Can you work these out from the model? Positions are in its coordinate system, mm. A direction names the side the tool comes from. Coordinates: 2 decimals unless noted, no trailing zeros. Order: outer loops, then holes, each group sorted by start corner. A loop starts at its lowest first (then second) coordinate and runs counter-clockwise, first axis right, second up. Notation, with made-up numbers: (-11.5, 48.5) -> (-6.5, 48.5) arc R13 cw to (-6.5, 58.5) -> close; hole circle Ø3 at (13, 6). An arc over 180 degrees is marked (long way). Answer as CSV lines item,"result".
Autodesk Inventor part; units mm, degrees
ref_plane "YZ Plane" through (0, 0, 0) normal (1, 0, 0) x (0, 1, 0)
ref_plane "XZ Plane" through (0, 0, 0) normal (0, 1, 0) x (-1, 0, 0)
ref_plane "XY Plane" through (0, 0, 0) normal (0, 0, 1) x (1, 0, 0)
sketch "Sketch1" plane through (0, 0, 0) normal (0, 1, 0) x (-1, 0, 0)
  line L0 (0, 0) -> (28, 0)
  line L1 (28, 0) -> (28, -6)
  line L2 (28, -6) -> (0, -6)
  line L3 (0, -6) -> (0, 0)
  dimension "d0" = 28
  dimension "d1" = 6
extrude "Extrusion1" add sketch "Sketch1" along normal blind 2.54
hole "Hole1" at (-25.5, 2.54, -2.952) direction (0, -1, 0) diameter 4 end through all
hole "Hole2" at (-2.5, 2.54, -2.952) direction (0, -1, 0) diameter 4 end through all
sketch "Sketch2" plane through (0, 0, 0) normal (1, 0, 0) x (0, 0, -1)
  circle A0 centre (-3.7852, -0.96) radius 3.5
  line L0 (-3.7852, 2.54) -> (0.6598, 2.54)
  line L1 (0, 2.54) -> (6, 2.54)
  line L2 (6, 0) -> (0, 0)
  line L3 (-0.4194, 0) -> (0, 0)
  line L4 (0, 0) -> (-0.4194, 0)
  line L5 (0.2994, 0) -> (-3.7852, 0)
  line L6 (-3.7852, 0) -> (-3.7852, 2.54)
  line L7 (-3.7852, 2.54) -> (0.2994, 2.54)
  line L8 (0.2994, 2.54) -> (0.2994, 0)
  line L9 (0.2994, 2.54) -> (-3.6886, 2.54)
  line L10 (-3.6886, 2.54) -> (-3.6886, 0)
  line L11 (-3.6886, 0) -> (0.2994, 0)
  line L12 (0.2994, 0) -> (0.2994, 2.54)
  dimension "d22" = 7
  dimension "d41" = 4.445
extrude "Extrusion2" add sketch "Sketch2" against normal blind 28
sketch "Sketch3" plane through (0, 2.54, 0) normal (0, 1, 0) x (1, 0, 0)
  line L0 (-28, 0) -> (-17.5, 0)
  line L1 (-17.5, 0) -> (-17.5, -12.7)
  line L2 (-17.5, -12.7) -> (-28, -12.7)
  line L3 (-28, -12.7) -> (-28, 0)
  line L4 (0, 0) -> (0, 6)
  line L5 (0, 0) -> (-10.5, 0)
  line L6 (-10.5, 0) -> (-10.5, -9.3969)
  line L7 (-10.5, -9.3969) -> (0, -9.3969)
  line L8 (0, -9.3969) -> (0, 0)
  dimension "d28" = 7
  dimension "d29" = 10.5
  dimension "d42" = 12.7
extrude "Extrusion3" cut sketch "Sketch3" against normal blind 28
hole "Hole3" at (-10.5, -0.96, 3.7852) direction (-1, 0, 0) diameter 3 end through all
properties part number "camera holderpt2"
Q1. Imagine slicing it at A-A (y = -0.96). List the corners of the cut face in (x, z) for me.
Solution:
outline,"(-17.5, 0.29) -> (-10.5, 0.29) -> (-10.5, 2.29) -> (-17.5, 2.29) -> close; (-17.5, 5.29) -> (-10.5, 5.29) -> (-10.5, 7.29) -> (-17.5, 7.29) -> close"
Q2. Imagine slicing it at C-C (y = 2.25). List the corners of the cut face in (x, z) for me, and give its area (3 significant figures).
Solution:
outline,"(-28, -6) -> (0, -6) -> (0, 0) -> (-10.5, 0) -> (-10.5, 5.18) -> (-17.5, 5.18) -> (-17.5, 0) -> (-28, 0) -> close; hole circle Ø4 at (-25.5, -2.95); hole circle Ø4 at (-2.5, -2.95)"
area,"179 mm2"
Q3. Imagine slicing it at D-D (x = -16). List the corners of the cut face in (y, z) for me, and give its area (3 significant figures).
Solution:
outline,"(0, -6) -> (2.54, -6) -> (2.54, 3.69) arc R3.5 ccw (long way) to (0, 0.42) -> close; hole circle Ø3 at (-0.96, 3.79)"
area,"50.0 mm2"
Q4. If I drill on line 1 (X direction, y = 1.75, z = -3); line 2 (Z direction, x = -2.5, y = 1.8); line 3 (Z direction, x = -21.5, y = 0.75), over which ranges is the centre line in solid material (lowest first)?
Solution:
line 1,"-28 to -27.5, -23.5 to -4.5, -0.5 to 0"
line 2,"-6 to -4.95, -0.95 to 0"
line 3,"-6 to 0"
Q5. We'd pull the mould along Z, two halves only. Please class faces 1 (the flat face through (-14, 1, -6)), 2 (the cylindrical face through (-14.049, 0.504, 4.11)), 3 (the flat face through (-10.5, 1, 4)): pulls with the +Z half, pulls with the -Z half, needs draft (parallel to the pull), parting line crosses it, or undercut.
Solution:
face 1,"pulls with the -Z half"
face 2,"undercut"
face 3,"needs draft"
Q6. For P1, Ø3, axis at x = -21.5, y = 0, coming from the +Z side; P2, Ø2, axis at y = -1, z = 3, coming from the +X side; P3, Ø5, axis at x = -19, z = -0.5, coming from the -Y side; P4, Ø5, axis at x = -2.5, z = -2.952, coming from the +Y side, each with a flat end and sliding along its axis, tell me the tip position at first contact or that it passes through.
Solution:
P1,"z = 0"
P2,"x = -10.5"
P3,"y = -3.61"
P4,"y = 2.54"
Q7. Which directions (+Z, -Z, +X, -X, +Y, -Y) give clear straight access to the entire face, cutting with the end or side of a thin tool? Please do faces 4 (the flat face through (-17.5, 1, 4)), 5 (the flat face through (-5, 1, 0)), 6 (the flat face through (0, 1, -3)).
Solution:
face 4,"+Z, -X, +Y, -Y"
face 5,"+Z, +X, +Y, -Y"
face 6,"+Z, -Z, +X, +Y, -Y"
Q8. Imagine slicing it at B-B (x = -2.5). List the corners of the cut face in (y, z) for me.
Solution:
outline,"(0, -6) -> (2.54, -6) -> (2.54, -4.95) -> (0, -4.95) -> close; (0, -0.95) -> (2.54, -0.95) -> (2.54, 0) -> (0, 0) -> close"
